Input: dimensioned drawing with shaded views. Units: mm. Origin: part minimum x, y, z. Give positions to 0.01 mm unless a question says otherwise; leave off trailing zeros. Write each loop counter-clockwise with the first axis right and the second up, starting at its lowest first coordinate (ties: lowest second). Pieces come first, ordered by that corner, then holes. Notation, with made-up numbers: (43.25, 3.25) -> (68.25, 3.25) arc R14 cw to (68.25, 29.25) -> close; hole circle Ø7 at (-8.5, -28). An arc over 180 degrees is marked (long way). Answer as a JSON object with one key per item and string values.
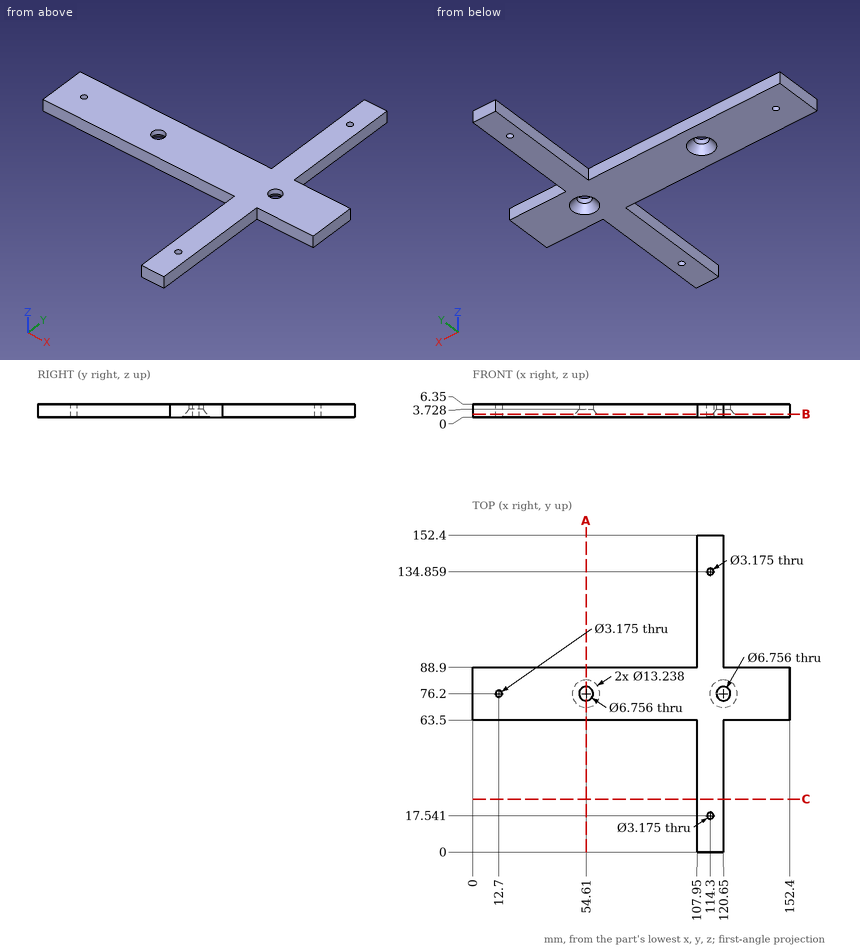
Q1. Cut plane C-C (y = 25.5). Return the cut outline in (x, z).
Values:
{"outline": "(107.95, 0) -> (120.65, 0) -> (120.65, 6.35) -> (107.95, 6.35) -> close"}
Q2. First-contact query: P1, Ø2, axis at x = 43.5, z = 5, coming from the +Y side; P2, Ø3, axis at y = 124.5, z = 2, coming from the +X side; P3, Ø2.5, axis at x = 114.3, y = 17.54, coming from the +Z side; P4, Ø1.5, axis at x = 37, z = 3, coming from the -Y side. Flat tips, straight axial feed; report the tip coordinate or a pass-through.
Values:
{"P1": "y = 88.9", "P2": "x = 120.65", "P3": "through", "P4": "y = 63.5"}
Q3. Material intervals for L1, parallel to X at y = 76.2, z = 4; L2, parallel to Y at x = 114.3, z = 4; L3, parallel to Y at x = 54.61, z = 5.1, sorted ascending. Write a range as from..to.
Values:
{"L1": "0..11.11, 14.29..51.23, 57.99..117.27, 124.03..152.4", "L2": "0..15.95, 19.13..133.27, 136.45..152.4", "L3": "63.5..72.82, 79.58..88.9"}
Q4. Cut plane B-B (z = 1.5). State how many separate pieces and enclosed holes the cut face has, and give its area (3 significant figures).
Values:
{"separate pieces": "1", "enclosed holes": "5", "area": "5,280 mm²"}
Q5. Cut plane A-A (x = 54.61). Return the cut outline in (y, z).
Values:
{"outline": "(63.5, 0) -> (69.58, 0) -> (72.82, 3.73) -> (72.82, 6.35) -> (63.5, 6.35) -> close; (79.58, 3.73) -> (82.82, 0) -> (88.9, 0) -> (88.9, 6.35) -> (79.58, 6.35) -> close"}
